For this review, take the finished solid that the model builds, in its own axes (mm). A direction names the side the tool comes from. Give positions to 0.01 mm unless a question says otherwise; leave off trailing zeros. Order: outer loops, then holes, each group sorted by start corner. A loop starts at its lowest first (then second) coordinate and runs counter-clockwise, first axis right, second up.
Item 1: Machinability: for faces 1 (the flat face through (0, -12, 0)), 2 (the cylindrical face through (-1.19, -7.07, -5.37)), which of the approach directions +Z, -Z, +X, -X, +Y, -Y give a long, thin tool a straight path to every point of the face, cutting with its end or side? Answer none if there is none.
Item 2: For probe 1 along Y at (x, z) = (6, -3); probe 2 along Z at (x, y) = (-2.5, -9.25); probe 3 along Z at (x, y) = (-0.25, -11), list the stretches that pass through material, from the lowest coordinate up.
Item 3: Consider section C-C (y = -8). Give the boundary of the cut face in (x, z), plus the area to 3 significant figures.
Item 4: Consider section A-A (x = 0). Give the boundary of the cut face in (y, z), plus the area to 3 significant figures.
Item 5: Consider section B-B (z = 0). Give the boundary of the cut face in (x, y).
Item 6: For P1, Ø3, axis at x = -6.5, z = 1.5, coming from the -Y side; P2, Ø1, axis at x = -1, y = -6.5, coming from the +Z side; P3, Ø6, axis at y = -3, z = -5, coming from the -X side; P4, Ø1, axis at y = -8.5, z = -4, coming from the +X side, all flat-tipped, find the tip position at first contact; note any pin that passes through.
```python
from build123d import *

# Parameters (mm, degrees)
F0_R     = 9
F1_DEPTH = 12
F3_R     = 2
F2_R     = 9
F2_R_2   = 5.5
F4_DEPTH = 10


with BuildPart() as f1:
    # F0 (on Front) → F1 (new body)
    with BuildSketch(Plane.XZ):
        Circle(F0_R)
    extrude(amount=F1_DEPTH)

    # F3
    f3_edges = [f1.edges().sort_by_distance(p)[0] for p in [
        (-9, 0, 0),
    ]]
    fillet(f3_edges, radius=F3_R)

    # F2 (on face) → F4 (cut)
    with BuildSketch(Plane.XZ.offset(12)):
        Circle(F2_R)
        Circle(F2_R_2, mode=Mode.SUBTRACT)
    extrude(amount=-F4_DEPTH, mode=Mode.SUBTRACT)


solid = f1.part
```
Resolved:
1. face 1: +Z, -Z, +X, -X, -Y
1. face 2: -Y
2. probe 1: y = -2 to 0
2. probe 2: z = -4.9 to 4.9
2. probe 3: z = -5.49 to 5.49
3. outline: circle Ø11 at (0, 0)
3. area: 95.0 mm2
4. outline: (-12, -5.5) - (-2, -5.5) - (-2, -9) arc R2 ccw to (0, -7) - (0, 7) arc R2 ccw to (-2, 9) - (-2, 5.5) - (-12, 5.5) - close
4. area: 144 mm2
5. outline: (-9, -2) - (-5.5, -2) - (-5.5, -12) - (5.5, -12) - (5.5, -2) - (9, -2) arc R2 ccw to (7, 0) - (-7, 0) arc R2 ccw to start
6. P1: stops at y = -12
6. P2: stops at z = 5.48
6. P3: stops at x = -8.73
6. P4: stops at x = 4.24
